Check sheet for the modelled part. Datum: model origin and axes. Units: mm. A direction names the side the tool comes from. Round coordinates to 2 decimals unless told otherwise and drop trailing zeros. Order: outer loops, then holes, each group sorted by start corner. A loop starts at its lowest first (then second) coordinate and runs counter-clockwise, first axis right, second up.
(1) Sectioned sample at D-D, the plane y = -77.5. Enter the section's corners in (x, z).
(2) Mould release check, pull along Y, two halves, no side actions. Record for faces 1 (the cylindrical face through (-68.828, -125.551, -63.795)), 2 (the cylindrical face through (15.13, -25.76, -34.48)), 3 (the cylindrical face through (-51.36, -81.103, -0.934)): released by +Y, released by -Y, zero draft, split by the parting line, or undercut.
(3) Sectioned sample at C-C, the plane y = -102. Enter the section's corners in (x, z), and give its area (3 significant figures).
(4) Depth check by flat-ended pin: pin 1 (8 mm diameter, centred on x = -28, y = -55.5, fed in from -Z); pin 2 (14 mm diameter, centred on x = -23, y = -74, fed in from -Z). Enter the tip coordinate at first touch or a pass-through.
(5) Thickness scan on probe 1 along Y at (x, z) = (-19, -22); probe 2 along X at (y, z) = (-98.5, 30); probe 3 along Y at (x, z) = (-72, 0). Record the ranges inside material, lowest first.
(6) Sectioned sample at A-A, the plane z = -23.5. Enter the section's corners in (x, y).
(7) Sectioned sample at B-B, the plane x = 21. Enter the section's corners in (y, z).
(8) Tool access check on faces 4 (the cylindrical face through (14.9, -49.3, 60.2)), 5 (the cylindrical face through (-35.92, -88.44, -3.27)), 6 (the flat face through (65.434, -25.044, 9.164)), 7 (the flat face through (0.649, -89, 30)). Record the directions out of +Z, -Z, +X, -X, +Y, -Y that give a thin tool (end or side, any length) a straight path to the whole face; none if there is none.
```python
from build123d import *

# Parameters (mm, degrees)
F0_W     = 203.2
F0_H     = 127
F1_DEPTH = 127
F3_DEPTH = 76.2
F4_SIZE2 = 101.6
F4_SIZE  = 76.2
F5_R     = 5.08
F6_R     = 15.24
F7_DEPTH = 50.8
F8_R     = 25.4
F9_DEPTH = 127


with BuildPart() as f1:
    # F0 (on Front) → F1 (new body)
    with BuildSketch(Plane.XZ):
        with Locations((0.6489251732, -1.8226355314)):
            Rectangle(F0_W, F0_H)
    extrude(amount=F1_DEPTH)

    # F2 (on face) → F3 (cut)
    with BuildSketch(Plane.XZ.offset(127)):
        Polygon((102.2489251732, 61.6773644686), (0.6489251732, 61.6773644686), (0.6489251732, -1.8226355314), (-37.4510748268, -1.8226355314), (-37.4510748268, -65.3226355314), (102.2489251732, -65.3226355314), align=None)
    extrude(amount=-F3_DEPTH, mode=Mode.SUBTRACT)

    # F4
    f4_edges = [f1.edges().sort_by_distance(p)[0] for p in [
        (102.248925, -25.4, 61.677364),
    ]]
    f4_side = f1.faces().sort_by_distance((-21.122503, -52.614286, 61.677364))[0]
    chamfer(f4_edges, length=F4_SIZE, length2=F4_SIZE2, reference=f4_side)

    # F5
    f5_edges = [f1.edges().sort_by_distance(p)[0] for p in [
        (-50.151075, -127, 61.677364),
        (-37.451075, 0, 61.677364),
        (26.048925, -25.4, 61.677364),
        (-100.951075, -63.5, 61.677364),
        (13.348925, -50.8, 61.677364),
        (0.648925, -88.9, 61.677364),
        (0.648925, -127, 29.927364),
        (0.648925, -88.9, -1.822636),
        (0.648925, -50.8, 29.927364),
        (-37.451075, -88.9, -1.822636),
        (-37.451075, -88.9, -65.322636),
        (-37.451075, -127, -33.572636),
        (-37.451075, -50.8, -33.572636),
        (-69.201075, -127, -65.322636),
        (-100.951075, -63.5, -65.322636),
        (-100.951075, 0, -1.822636),
        (-100.951075, -127, -1.822636),
        (0.648925, 0, -65.322636),
        (32.398925, -50.8, -65.322636),
        (-18.401075, -50.8, -1.822636),
        (-18.401075, -127, -1.822636),
    ]]
    fillet(f5_edges, radius=F5_R)

    # F6 (on face) → F7 (cut, through all)
    with BuildSketch(Plane.XZ.offset(50.8)):
        with Locations((18.4289251732, -19.6026355314)):
            Circle(F6_R)
    extrude(amount=-F7_DEPTH, mode=Mode.SUBTRACT)

    # F8 (on face) → F9 (cut, through all)
    with BuildSketch(Plane.XY.offset(61.6773644686)):
        with Locations((-63.0807951093, -58.5683807731)):
            Circle(F8_R)
    extrude(amount=-F9_DEPTH, mode=Mode.SUBTRACT)


solid = f1.part
```
Derived:
1. outline: (-100.95, -60.24) arc R5.08 ccw to (-95.87, -65.32) - (-80.01, -65.32) - (-80.01, 61.68) - (-95.87, 61.68) arc R5.08 ccw to (-100.95, 56.6) - close; (-46.15, -65.32) - (-42.53, -65.32) arc R5.08 ccw to (-37.45, -60.24) - (-37.45, -6.9) arc R5.08 cw to (-32.37, -1.82) - (-4.43, -1.82) arc R5.08 ccw to (0.65, 3.26) - (0.65, 56.6) arc R5.08 ccw to (-4.43, 61.68) - (-46.15, 61.68) - close
2. face 1: released by -Y
2. face 2: zero draft
2. face 3: undercut
3. outline: (-100.95, -60.24) arc R5.08 ccw to (-95.87, -65.32) - (-42.53, -65.32) arc R5.08 ccw to (-37.45, -60.24) - (-37.45, -6.9) arc R5.08 cw to (-32.37, -1.82) - (-4.43, -1.82) arc R5.08 ccw to (0.65, 3.26) - (0.65, 56.6) arc R5.08 ccw to (-4.43, 61.68) - (-95.87, 61.68) arc R5.08 ccw to (-100.95, 56.6) - close
3. area: 10,500 mm2
4. pin 1: stops at z = -4.33
4. pin 2: stops at z = -1.82
5. probe 1: y = -50.8 to 0
5. probe 2: x = -100.95 to 0.65
5. probe 3: y = -127 to -82.35, -34.79 to 0
6. outline: (-100.95, -121.92) arc R5.08 ccw to (-95.87, -127) - (-42.53, -127) arc R5.08 ccw to (-37.45, -121.92) - (-37.45, -55.88) arc R5.08 cw to (-32.37, -50.8) - (3.7, -50.8) - (3.7, 0) - (-95.87, 0) arc R5.08 ccw to (-100.95, -5.08) - close; (33.16, -50.8) - (89.93, -50.8) - (89.93, 0) - (33.16, 0) - close; hole circle Ø50.8 at (-63.08, -58.57)
7. outline: (-50.8, -60.24) arc R5.08 ccw to (-45.72, -65.32) - (-5.08, -65.32) arc R5.08 ccw to (0, -60.24) - (0, -34.62) - (-50.8, -34.62) - close; (-50.8, -4.58) - (0, -4.58) - (0, 56.6) arc R5.08 ccw to (-5.08, 61.68) - (-45.72, 61.68) arc R5.08 ccw to (-50.8, 56.6) - close
8. face 4: +Z, +X, -Y
8. face 5: -Z, +X, -Y
8. face 6: +Z, +X, +Y, -Y
8. face 7: +Z, -Z, +X, -Y
